from build123d import *

# Parameters (mm, degrees)
SKETCH2_R          = 2.5
CUT_EXTRUDE1_DEPTH = 20.261360284


with BuildPart() as part:
    # Sketch1 → Revolve1 (revolve)
    with BuildSketch(Plane.XY, mode=Mode.PRIVATE) as revolve1_sk:
        with BuildLine():
            Line((-6, 7), (-4, 7))
            Line((-4, 7), (-4, 5))
            ThreePointArc((-4, 5), (-6.403124237, 0), (-4, -5))
            Line((-4, -5), (-4, -7))
            Line((-4, -7), (-6, -7))
            Line((-6, -7), (-6, -8.5))
            Line((-6, -8.5), (0, -8.5))
            Line((0, -8.5), (0, 8.5))
            Line((0, 8.5), (-6, 8.5))
            Line((-6, 8.5), (-6, 7))
        make_face()
    revolve(revolve1_sk.sketch.rotate(Axis((0, 16.114211291, 0), (0, -1, 0)), 270), axis=Axis((0, 16.114211291, 0), (0, -1, 0)))

    # Sketch2 → Cut-Extrude1 (cut, through all)
    with BuildSketch(Plane(origin=(0, 8.5, 0), x_dir=(1, 0, 0), z_dir=(0, 1, 0))):
        with Locations(Location((0, 0, 0), (0, 0, 270))):
            Circle(SKETCH2_R)
    extrude(amount=-CUT_EXTRUDE1_DEPTH, mode=Mode.SUBTRACT)


solid = part.part
Geometry check sheet. Reference: the model listing, model coordinates, mm. A direction names the side the tool comes from. Give positions to 0.01 mm unless a question says otherwise; leave off trailing zeros. Order: outer loops, then holes, each group sorted by start corner. A loop starts at its lowest first (then second) coordinate and runs counter-clockwise, first axis right, second up. Notation, with made-up numbers: (58.5, 32.5) - (67.5, 32.5) arc R6 cw to (67.5, 43.5) - close; hole circle Ø1 at (-15.5, -9.5). An arc over 180 degrees is marked (long way). Answer as a JSON object with one key per item and string values.
(1) Cross-section at D-D (y = 0). Record the cut outline in (x, z).
Report:
{"outline": "circle Ø12.81 at (0, 0); hole circle Ø5 at (0, 0)"}
(2) Cross-section at C-C (x = -4.5). Record the cut outline in (y, z), then the cut area to 3 significant figures.
Report:
{"outline": "(-8.5, -3.97) - (-7, -3.97) - (-7, 3.97) - (-8.5, 3.97) - close; circle Ø9.11 at (0, 0); (7, -3.97) - (8.5, -3.97) - (8.5, 3.97) - (7, 3.97) - close", "area": "89.0 mm^2"}
(3) Cross-section at B-B (z = -1.25). Record the cut outline in (x, y), then the cut area to 3 significant figures.
Report:
{"outline": "(-5.87, -8.5) - (-2.17, -8.5) - (-2.17, 8.5) - (-5.87, 8.5) - (-5.87, 7) - (-3.8, 7) - (-3.8, 5) arc R6.28 ccw to (-3.8, -5) - (-3.8, -7) - (-5.87, -7) - close; (2.17, -8.5) - (5.87, -8.5) - (5.87, -7) - (3.8, -7) - (3.8, -5) arc R6.28 ccw to (3.8, 5) - (3.8, 7) - (5.87, 7) - (5.87, 8.5) - (2.17, 8.5) - close", "area": "103 mm^2"}
(4) Depth check by flat-ended pin: pin 1 Ø6.5 at (x, z) = (0, 0) entering from +Y; pin 2 Ø4 at (x, y) = (2, -1) entering from +Z; pin 3 Ø6 at (x, y) = (0, 3.5) entering from -Z; pin 4 Ø4 at (y, z) = (3.5, 1) entering from -X. Enter the tip coordinate at first touch or a pass-through.
Report:
{"pin 1": "y = 8.5", "pin 2": "z = 6.4", "pin 3": "z = -6.38", "pin 4": "x = -6.19"}
(5) Tool access check on faces 4 (the cylindrical face through (3.905, -6.014, -0.867)), 5 (the cylindrical face through (-1.802, 7.74, 5.723)), 6 (the flat face through (0, -8.5, 3)), 7 (the cylindrical face through (-1.802, -7.76, 5.723)). Record the directions out of +Z, -Z, +X, -X, +Y, -Y that give a thin tool (end or side, any length) a straight path to the whole face; none if there is none.
Report:
{"face 4": "none", "face 5": "+Y", "face 6": "+Z, -Z, +X, -X, -Y", "face 7": "-Y"}
(6) Draft check along Z on faces 1 (the flat face through (3.92, -7, 1.42)), 2 (the cylindrical face through (3.905, 5.986, -0.867)), 3 (the cylindrical face through (-2.44, 0.12, -0.54)). Enter one of: released by +Z, released by -Z, zero draft, split by the parting line, or undercut.
Report:
{"face 1": "zero draft", "face 2": "split by the parting line", "face 3": "undercut"}
(7) Cross-section at A-A (x = 2.25). Record the cut outline in (y, z), then the cut area to 3 significant figures.
Report:
{"outline": "(-8.5, -5.56) - (-7, -5.56) - (-7, -3.31) - (-5, -3.31) arc R5.99 ccw to (5, -3.31) - (7, -3.31) - (7, -5.56) - (8.5, -5.56) - (8.5, -1.09) - (-8.5, -1.09) - close; (-8.5, 1.09) - (8.5, 1.09) - (8.5, 5.56) - (7, 5.56) - (7, 3.31) - (5, 3.31) arc R5.99 ccw to (-5, 3.31) - (-7, 3.31) - (-7, 5.56) - (-8.5, 5.56) - close", "area": "127 mm^2"}
(8) Material ranges on line 1 (Y direction, x = -3.5, z = 4.5); line 2 (Y direction, x = 1.5, z = -5); line 3 (Z direction, x = 2, y = -2.25), recorded low to high.
Report:
{"line 1": "-8.5 to -7, -2.92 to 2.92, 7 to 8.5", "line 2": "-8.5 to -7, -3.71 to 3.71, 7 to 8.5", "line 3": "-5.65 to -1.5, 1.5 to 5.65"}
